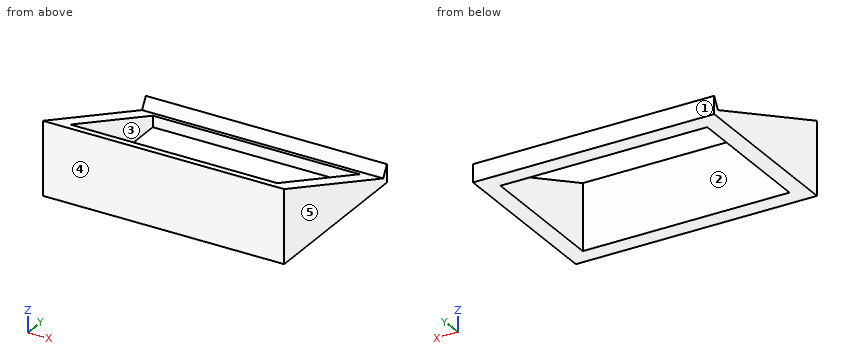
```python
from build123d import *

# Parameters (mm, degrees)
F0_W     = 177.8
F0_H     = 127
F1_DEPTH = 50.8
F3_DEPTH = 2514.6
F4_DEPTH = 3.175
F6_DEPTH = 2514.6


with BuildPart() as f1:
    # F0 (on Top) → F1 (new body)
    with BuildSketch(Plane.XY):
        Rectangle(F0_W, F0_H)
    extrude(amount=F1_DEPTH)

    # F2 (on face) → F3 (cut)
    with BuildSketch(Plane(origin=(-88.9, 0, 0), x_dir=(0, -1, 0), z_dir=(-1, 0, 0))):
        Polygon((-63.5, 9.9646151066), (-58.8191700766, 1.8723319694), (63.5, 50.8), (-63.5, 50.8), align=None)
    extrude(amount=-F3_DEPTH, mode=Mode.SUBTRACT)

    # F4 (add): a face of the model
    f4_faces = [f1.faces().sort_by_distance(p)[0] for p in [
        (0, 0, 0),
    ]]
    extrude(f4_faces, amount=F4_DEPTH)

    # F5 (on face) → F6 (cut)
    with BuildSketch(Plane(origin=(0, 0, -3.175), x_dir=(1, 0, 0), z_dir=(0, 0, -1))):
        Polygon((-76.2, -50.8), (76.2, -50.8), (76.2, 0), (76.2, 50.8), (0, 50.8), (-76.2, 50.8), align=None)
    extrude(amount=-F6_DEPTH, mode=Mode.SUBTRACT)


solid = f1.part
```
Design review of the part built by this model. Coordinates are the model's own, in mm. Face numbers are marked on the shaded views. A direction names the side the tool comes from. Give positions to 0.01 mm unless a question says otherwise; leave off trailing zeros. Write each loop counter-clockwise with the first axis right and the second up, starting at its lowest first coordinate (ties: lowest second). Pieces come first, ordered by that corner, then holes.
(1) Add section A-A (y = 16.5). Give the boundary of the cut face in (x, z) (3 decimals).
Checked values:
outline: (-88.9, -3.175) - (-76.2, -3.175) - (-76.2, 18.8) - (-88.9, 18.8) - close; (76.2, -3.175) - (88.9, -3.175) - (88.9, 18.8) - (76.2, 18.8) - close
(2) Wall thickness on line 1 along X through (y, z) = (-41, 37); line 2 along Y through (x, z) = (-1.5, 1.5); line 3 along Y through (x, z) = (45, 41.5): over which ranges is each line inside the solid? List them lowest first.
Checked values:
line 1: x = -88.9 to -76.2, 76.2 to 88.9
line 2: y = -63.5 to -50.8, 50.8 to 63.5
line 3: y = -63.5 to -50.8
(3) Add section B-B (x = -61). Give the boundary of the cut face in (y, z) (3 decimals), and give its area (3 significant figures).
Checked values:
outline: (-63.5, -3.175) - (-50.8, -3.175) - (-50.8, 45.72) - (-63.5, 50.8) - close; (50.8, -3.175) - (63.5, -3.175) - (63.5, 9.965) - (58.819, 1.872) - (50.8, 5.08) - close
area: 749 mm2
(4) Mouldability with a two-part tool opening along Y and no side actions: class the marked faces 3, 4 and 5 as +Y half, -Y half, draft (parallel to the pull), parting line (faces both ways), or undercut.
Checked values:
face 3: undercut
face 4: -Y half
face 5: draft
(5) Tool access review of the marked faces 1 and 2: name each direction out of +Z, -Z, +X, -X, +Y, -Y from which nothing blocks a thin tool from reaching the whole face with its end or side.
Checked values:
face 1: +Z, -Z, +X, -X, +Y
face 2: +Z, -Z
(6) Add section C-C (z = 38). Give the boundary of the cut face in (x, y), and give its area (3 significant figures).
Checked values:
outline: (-88.9, -63.5) - (88.9, -63.5) - (88.9, -31.5) - (76.2, -31.5) - (76.2, -50.8) - (-76.2, -50.8) - (-76.2, -31.5) - (-88.9, -31.5) - close
area: 2,750 mm2
(7) Add section D-D (y = -35.5). Give the boundary of the cut face in (x, z) (3 decimals).
Checked values:
outline: (-88.9, -3.175) - (-76.2, -3.175) - (-76.2, 39.6) - (-88.9, 39.6) - close; (76.2, -3.175) - (88.9, -3.175) - (88.9, 39.6) - (76.2, 39.6) - close
(8) Clearance check with flat-ended pins moving along their axes: pin 1 Ø10 at (x, z) = (14.5, 27.5) entering from +Y; pin 2 Ø10 at (y, z) = (11, 22.5) entering from -X. State where each tip first meets the part, or that it passes through.
Checked values:
pin 1: stops at y = -50.8
pin 2: stops at x = -88.9
